Source: CAD feature listing. Evaluate the final solid. Frame: model axes, mm. Give positions to 0.01 mm unless a question says otherwise; leave off trailing zeros. Order: outer loops, then holes, each group sorted by start corner. A loop starts at its lowest first (then second) coordinate and runs counter-clockwise, first axis right, second up. Notation, with made-up numbers: (27.25, -24) -> (64.25, -24) arc R13 ccw to (64.25, -2) -> close; hole circle Ø6 at (-38.5, -6.75). An arc over 180 degrees is marked (long way). Use CSV: the item, a comma, the result in double quotes.
```python
from build123d import *

# Parameters (mm, degrees)
F0_W     = 42
F0_H     = 42
F1_DEPTH = 1
F2_D     = 29
F3_D     = 2.8
F4_R     = 5


with BuildPart() as f1:
    # F0 (on Front) → F1 (new body)
    with BuildSketch(Plane.XZ):
        with Locations((-12.5967783645, -3.5383866066)):
            Rectangle(F0_W, F0_H)
    extrude(amount=F1_DEPTH)

    # F2 (through all)
    with Locations(Plane(origin=(0, 0, 0), x_dir=(1, 0, 0), z_dir=(0, 1, 0))):
        with Locations((-12.5967783645, 3.5383866066)):
            Hole(F2_D / 2)

    # F3 (through all)
    with Locations(Plane(origin=(0, 0, 0), x_dir=(1, 0, 0), z_dir=(0, 1, 0))):
        with Locations((-28.0967783645, -11.9616133934), (2.9032216355, -11.9616133934), (2.9032216355, 19.0383866066), (-28.0967783645, 19.0383866066)):
            Hole(F3_D / 2)

    # F4
    f4_edges = [f1.edges().sort_by_distance(p)[0] for p in [
        (-33.596778, -0.5, 17.461613),
        (-33.596778, -0.5, -24.538387),
        (8.403222, -0.5, 17.461613),
        (8.403222, -0.5, -24.538387),
    ]]
    fillet(f4_edges, radius=F4_R)


solid = f1.part
```
1. Pin query (flat end, axial travel): P1, Ø1, axis at x = -4.5, z = -15.5, coming from the +Y side. Return the tip coordinate at first contact, or that it passes through.
Answer below:
P1,"stops at y = 0"
2. Mould query, pull axis Z, two halves, no side actions, for faces 1 (the cylindrical face through (6.9, -0.51, -23.11)), 2 (the flat face through (-12.8, -0.5, 17.462)), 3 (the cylindrical face through (2.15, -0.51, -20.22)), 4 (the cylindrical face through (-29.43, -0.51, 11.54)). Classes: released by +Z, released by -Z, zero draft, split by the parting line, or undercut.
Answer below:
face 1,"released by -Z"
face 2,"released by +Z"
face 3,"undercut"
face 4,"undercut"
3. Section query C-C on x = -28. Return loops of the section in (y, z), plus the area to 3 significant figures.
Answer below:
outline,"(-1, -24.54) -> (0, -24.54) -> (0, -20.44) -> (-1, -20.44) -> close; (-1, -17.64) -> (0, -17.64) -> (0, 10.56) -> (-1, 10.56) -> close; (-1, 13.36) -> (0, 13.36) -> (0, 17.46) -> (-1, 17.46) -> close"
area,"36.4 mm²"
4. Section query A-A on x = -2.5. Return loops of the section in (y, z).
Answer below:
outline,"(-1, -24.54) -> (0, -24.54) -> (0, -13.95) -> (-1, -13.95) -> close; (-1, 6.87) -> (0, 6.87) -> (0, 17.46) -> (-1, 17.46) -> close"
5. Section query D-D on y = -0.25. Return loops of the section in (x, z), plus the area to 3 significant figures.
Answer below:
outline,"(-33.6, -19.54) arc R5 ccw to (-28.6, -24.54) -> (3.4, -24.54) arc R5 ccw to (8.4, -19.54) -> (8.4, 12.46) arc R5 ccw to (3.4, 17.46) -> (-28.6, 17.46) arc R5 ccw to (-33.6, 12.46) -> close; hole circle Ø2.8 at (-28.1, -19.04); hole circle Ø2.8 at (-28.1, 11.96); hole circle Ø29 at (-12.6, -3.54); hole circle Ø2.8 at (2.9, -19.04); hole circle Ø2.8 at (2.9, 11.96)"
area,"1,060 mm²"
6. Section query B-B on z = -3. Return loops of the section in (x, y), plus the area to 3 significant figures.
Answer below:
outline,"(-33.6, -1) -> (-27.09, -1) -> (-27.09, 0) -> (-33.6, 0) -> close; (1.89, -1) -> (8.4, -1) -> (8.4, 0) -> (1.89, 0) -> close"
area,"13.0 mm²"
7. Ray query, line 1 along Z through (x, y) = (-12.5, -0.9); line 2 along X through (y, z) = (-0.8, -20); line 3 along X through (y, z) = (-0.85, 13). Return the intervals inside material, ascending.
Answer below:
line 1,"z = -24.54 to -18.04, 10.96 to 17.46"
line 2,"x = -33.58 to -29.11, -27.08 to 1.89, 3.92 to 8.38"
line 3,"x = -33.57 to -29.04, -27.16 to 1.96, 3.84 to 8.37"
